```python
from build123d import *

# Parameters (mm, degrees)
SKETCH_10_W       = 200
SKETCH_10_H       = 150
EXTRUDE_401_DEPTH = 40
SKETCH_11_W       = 100
SKETCH_11_H       = 100
EXTRUDE_558_DEPTH = 1
SKETCH_12_W       = 60
SKETCH_12_H       = 60
EXTRUDE_709_DEPTH = 60
SKETCH_13_W       = 14
SKETCH_13_H       = 5
EXTRUDE_893_DEPTH = 3


with BuildPart() as part:
    # Эскиз10 → Extrude 401 (new body)
    with BuildSketch(Plane(origin=(0, 0, 0), x_dir=(1, 0, 0), z_dir=(0, 1, 0))):
        with Locations((50.389807825, -40.872183235)):
            Rectangle(SKETCH_10_W, SKETCH_10_H)
    extrude(amount=EXTRUDE_401_DEPTH)

    # Эскиз11 → Extrude 558 (add)
    with BuildSketch(Plane(origin=(0, 40, 0), x_dir=(1, 0, 0), z_dir=(0, 1, 0))):
        with Locations((30.223196857, -36.076377212)):
            Rectangle(SKETCH_11_W, SKETCH_11_H)
    extrude(amount=EXTRUDE_558_DEPTH)

    # Эскиз12 → Extrude 709 (add)
    with BuildSketch(Plane(origin=(0, 41, 0), x_dir=(1, 0, 0), z_dir=(0, 1, 0))):
        with Locations((25.734840207, -30)):
            Rectangle(SKETCH_12_W, SKETCH_12_H)
    extrude(amount=EXTRUDE_709_DEPTH)

    # Эскиз13 → Extrude 893 (add)
    with BuildSketch(Plane(origin=(0, 41, 0), x_dir=(1, 0, 0), z_dir=(0, 1, 0))):
        with Locations((2.012297913, -74.500076324)):
            Rectangle(SKETCH_13_W, SKETCH_13_H)
    extrude(amount=EXTRUDE_893_DEPTH)


solid = part.part
```
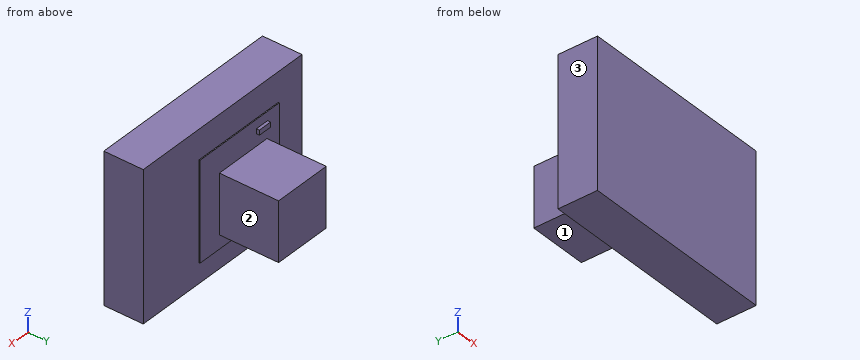
Build history of the part. All positions in model axes, mm. Face numbers are marked on the shaded views. A direction names the side the tool comes from. Coordinates: 2 decimals unless noted, no trailing zeros. Order: outer loops, then holes, each group sorted by start corner. A loop starts at its lowest first (then second) coordinate and runs counter-clockwise, first axis right, second up. Notation, with made-up numbers: (-39, 44.25) -> (-30, 44.25) arc R24 cw to (-30, 65.25) -> close; hole circle Ø2 at (53, -27.5). An arc over 180 degrees is marked (long way). Answer in a Markdown table with one row per item. Add a question column.
Q1. Band-saw the part on C-C, the plane y = 78. List the corners of the cut face in (x, z).
Q2. Wall check: line 1 along Z through (x, y) = (32.5, 70.5); line 2 along X through (y, z) = (93, 13); line 3 along Y through (x, z) = (108.5, 100). Give the ranges that are in metal, low to high. Write a range as [from, to].
Q3. Band-saw the part on D-D, the plane z = -10. List the corners of the cut face in (x, y).
Q4. Which spindle directions (+Z, -Z, +X, -X, +Y, -Y) get a long thin tool onto all of the face, cutting with end or side? Do the marked faces 1, 2 and 3. Say none if no direction does.
Q5. Band-saw the part on A-A, the plane z = 26. List the corners of the cut face in (x, y).
Q6. Drop flat-ended pins along their axis: pin 1 (1 mm diameter, centred on x = 73.5, z = 57.5, fed in from -Y); pin 2 (0.9 mm diameter, centred on y = 42.5, z = 75.5, fed in from +X); pin 3 (5.5 mm diameter, centred on x = 0.5, z = 74.5, fed in from +Y); pin 4 (1 mm diameter, centred on x = 77.5, z = 89.5, fed in from +Y). Give the stop position or say it passes through.
Q7. Band-saw the part on B-B, the plane x = 67.5. List the corners of the cut face in (y, z), then the cut area to 3 significant figures.
Answers follow:
| question | item | result |
|---|---|---|
| 1 | outline | (-4.27, 0) -> (55.73, 0) -> (55.73, 60) -> (-4.27, 60) -> close |
| 2 | line 1 | [0, 60] |
| 2 | line 2 | [-4.27, 55.73] |
| 2 | line 3 | [0, 40] |
| 3 | outline | (-49.61, 0) -> (150.39, 0) -> (150.39, 40) -> (80.22, 40) -> (80.22, 41) -> (-19.78, 41) -> (-19.78, 40) -> (-49.61, 40) -> close |
| 4 | face 1 | -Z, +X, -X, +Y |
| 4 | face 2 | +Z, -Z, +X, +Y |
| 4 | face 3 | +Z, -Z, -X, +Y, -Y |
| 5 | outline | (-49.61, 0) -> (150.39, 0) -> (150.39, 40) -> (80.22, 40) -> (80.22, 41) -> (55.73, 41) -> (55.73, 101) -> (-4.27, 101) -> (-4.27, 41) -> (-19.78, 41) -> (-19.78, 40) -> (-49.61, 40) -> close |
| 6 | pin 1 | y = 0 |
| 6 | pin 2 | x = 9.01 |
| 6 | pin 3 | y = 44 |
| 6 | pin 4 | y = 40 |
| 7 | outline | (0, -34.13) -> (40, -34.13) -> (40, -13.92) -> (41, -13.92) -> (41, 86.08) -> (40, 86.08) -> (40, 115.87) -> (0, 115.87) -> close |
| 7 | area | 6,100 mm^2 |
